```python
from build123d import *

# Parameters (mm, degrees)
SKETCH1_R           = 63.5
SKETCH2_R           = 50.8
SHELL1_T            = -10
SKETCH3_W           = 19.05
SKETCH3_H           = 6.858
BOSS_EXTRUDE1_DEPTH = 55.88
FILLET2_R           = 2
FILLET3_R           = 5


with BuildPart() as part:
    # Sketch1 → Loft1 section 0
    with BuildSketch(Plane.XY):
        Circle(SKETCH1_R)
    # Sketch2 → Loft1 section 1
    with BuildSketch(Plane.XY.offset(25.4)):
        Circle(SKETCH2_R)
    loft()

    # Shell1
    shell1_openings = [part.faces().sort_by_distance(p)[0] for p in [
        (0, 0, 0),
    ]]
    offset(amount=SHELL1_T, openings=shell1_openings, kind=Kind.INTERSECTION)

    # Sketch3 → Boss-Extrude1 (add)
    with BuildSketch(Plane.XY.offset(25.4)):
        with Locations((-12.7, 0)):
            Rectangle(SKETCH3_W, SKETCH3_H)
    extrude(amount=BOSS_EXTRUDE1_DEPTH)

    # Fillet2
    fillet2_edges = [part.edges().sort_by_distance(p)[0] for p in [
        (-22.225, 0, 81.28),
        (-12.7, -3.429, 81.28),
        (-3.175, 0, 81.28),
        (-12.7, 3.429, 81.28),
    ]]
    fillet(fillet2_edges, radius=FILLET2_R)

    # Fillet3
    fillet3_edges = [part.edges().sort_by_distance(p)[0] for p in [
        (-22.225, 0, 25.4),
        (-12.7, -3.429, 25.4),
        (-3.175, 0, 25.4),
        (-12.7, 3.429, 25.4),
    ]]
    fillet(fillet3_edges, radius=FILLET3_R)


solid = part.part
```
Geometry: final body of the model. Coordinates: model frame, mm. A direction names the side the tool comes from. Round coordinates to 2 decimals unless told otherwise and drop trailing zeros. Write each loop counter-clockwise with the first axis right and the second up, starting at its lowest first coordinate (ties: lowest second). Pieces come first, ordered by that corner, then holes. Notation, with made-up numbers: M 76,-15 L 107,-15 A20 ccw 107,15 Z; hole C -20,-33.5 d1. An arc over 180 degrees is marked long. Answer in a Markdown table with one row per item. Add a question column.
(1) Draft query along X for faces 1 (the face through (-12.497, -4.855, 26.904)), 2 (the face through (42.92, 13.51, 14.65)), 3 (the face through (-22.225, 0, 54)). Return one class per face: pulls with the +X half, pulls with the -X half, needs draft (parallel to the pull), parting line crosses it, or undercut.
(2) Cut plane C-C, the plane z = 22. Return the cut outline in (x, y), then the cut area to 3 significant figures.
(3) Reachability of faces 4 (the face through (-13, -3.429, 54)), 5 (the face through (-13, 3.429, 54)), 6 (the face through (-1, 1, 15.4)), 7 (the face through (9, 52, 0)), 8 (the face through (-3.175, 0, 54)) from +Z, -Z, +X, -X, +Y, -Y: full face, straight path, thin tool, end or side. Return the list, or none.
(4) Contact query for flat-ended pins moving along their axis: pin 1 (5.5 mm diameter, centred on y = -0.5, z = 57.5, fed in from +X) (3 decimals); pin 2 (1 mm diameter, centred on x = 12, y = -14.5, fed in from +Z); pin 3 (12 mm diameter, centred on x = 49, z = 20, fed in from -Y). Output: stop coordinate, or through.
(5) Cut plane A-A, the plane x = 0. Return the cut outline in (y, z), then the cut area to 3 significant figures.
(6) Cut plane B-B, the plane z = 63.5. Return the cut outline in (x, y) (3 decimals).
(7) Ray query, L1, parallel to Y at x = -12.5, z = 71.5; L2, parallel to Z at x = -37, y = -8; L3, parallel to X at y = 0, z = 57 (3 decimals). Return the intervals inside material, ascending.
Established:
| question | item | result |
|---|---|---|
| 1 | face 1 | needs draft |
| 1 | face 2 | undercut |
| 1 | face 3 | pulls with the -X half |
| 2 | outline | C 0,0 d105 |
| 2 | area | 8,660 mm² |
| 3 | face 4 | +Z, +X, -X, -Y |
| 3 | face 5 | +Z, +X, -X, +Y |
| 3 | face 6 | -Z |
| 3 | face 7 | -Z, +X, -X, +Y, -Y |
| 3 | face 8 | +Z, +X, +Y, -Y |
| 4 | pin 1 | x = -3.175 |
| 4 | pin 2 | z = 25.4 |
| 4 | pin 3 | y = -33.27 |
| 5 | outline | M -63.5,0 L -52.32,0 L -44.62,15.4 L 44.62,15.4 L 52.32,0 L 63.5,0 L 50.8,25.4 L 8.43,25.4 A5 cw 6.6,25.74 L -6.6,25.74 A5 cw -8.43,25.4 L -50.8,25.4 Z |
| 5 | area | 1,420 mm² |
| 6 | outline | M -22.225,-3.429 L -3.175,-3.429 L -3.175,3.429 L -22.225,3.429 Z |
| 7 | L1 | -3.43 to 3.43 |
| 7 | L2 | 15.4 to 25.4 |
| 7 | L3 | -22.225 to -3.175 |
